Design review of the part built by this model. Coordinates are the model's own, in mm. Face numbers are marked on the shaded views. A direction names the side the tool comes from. Coordinates: 2 decimals unless noted, no trailing zeros. Write each loop counter-clockwise with the first axis right and the second up, starting at its lowest first coordinate (ties: lowest second). Pieces come first, ordered by that corner, then holes.
Q1. Take a section at D-D, the plane x = 7. Write out the cut boundary in (y, z), plus the area to 3 significant figures.
Q2. Take a section at C-C, the plane y = 207. Write out the cut boundary in (x, z), plus the area to 3 significant figures.
Q3. Take a section at B-B, the plane x = 63. Write out the cut boundary in (y, z), plus the area to 3 significant figures.
Q4. For the marked faces 1 and 2, list the 3-axis set-ups (+Z, -Z, +X, -X, +Y, -Y) from which the entire face can be reached by the end or side of a thin tool; tool diameter is ignored.
Q5. For L1, parallel to Y at x = 87, z = -179.5; L2, parallel to Y at x = 46, z = -109; L3, parallel to X at y = 98, z = -88, list the stretches that pass through material, from the lowest coordinate up.
Q6. The part is to be moulded in two halves that separate along Y. For the marked faces 3, 4 and 5, say which applies: released by +Y, released by -Y, zero draft, split by the parting line, or undercut.
Q7. Take a section at A-A, the plane y = 36. Write out the cut boundary in (x, z).
Q8. For pin 1 Ø2 at (x, y) = (40, 225) entering from -Z; pin 2 Ø4 at (x, y) = (127.5, 58.5) entering from -Z; pin 3 Ø8 at (x, y) = (155, 320.5) entering from +Z, all flat-tipped, find the tip position at first contact; note any pin that passes through.
from build123d import *

# Parameters (mm, degrees)
BOSS_EXTRUDE1_DEPTH      = 254
BOSS_EXTRUDE2_DEPTH      = 165.1
BOSS_EXTRUDE2_DEPTH_BACK = 50.8
SKETCH16_R               = 20.3962
SKETCH17_R               = 25.4762
BOSS_EXTRUDE3_DEPTH      = 10.16
FILLET1_R                = 2.54
CUT_EXTRUDE5_DEPTH       = 518.859576594
CUT_EXTRUDE14_DEPTH      = 516.224718622
CUT_EXTRUDE16_DEPTH      = 488.341428789


with BuildPart() as part:
    # Sketch2 → Boss-Extrude1 (new body)
    with BuildSketch(Plane(origin=(0, 0, 0), x_dir=(1, 0, 0), z_dir=(0, 1, 0))):
        Polygon((0, 0), (130.302, 0), (154.729351402, 205.052140948), (-52.123869843, 143.209155408), align=None)
    extrude(amount=BOSS_EXTRUDE1_DEPTH)

    # Sketch16 → Boss-Extrude2 (add, two sides: drawn at the far end of the back side and taken through both)
    with BuildSketch(Plane(origin=(141.332693429, 246.526276938, 16.836612147), x_dir=(0.11829111292954252, 0, -0.9929789587911166), z_dir=(0.4964894793955593, 0.8660254037844382, 0.059145556464771376)).offset(-BOSS_EXTRUDE2_DEPTH_BACK)):
        with Locations(Location((59.539258978, 48.389402794, 0), (0, 0, 95.890220986))):
            Circle(SKETCH16_R)
    extrude(amount=BOSS_EXTRUDE2_DEPTH + BOSS_EXTRUDE2_DEPTH_BACK)

    # Sketch17 → Boss-Extrude3 (add)
    with BuildSketch(Plane(origin=(223.303106477, 389.507071103, 26.601543519), x_dir=(0.8680427390684899, -0.49533563558134813, -0.0338291482851031), z_dir=(0.49648947939555943, 0.866025403784438, 0.0591455564647714))):
        with Locations(Location((-39.824375463, 65.578020566, 0), (0, 0, 178.057961601))):
            Circle(SKETCH17_R)
    extrude(amount=-BOSS_EXTRUDE3_DEPTH)

    # Fillet1
    fillet1_edges = [part.edges().sort_by_distance(p)[0] for p in [
        (201.384117467, 394.758696828, -38.077767579),
        (210.835574876, 401.03092525, -37.476848726),
    ]]
    fillet(fillet1_edges, radius=FILLET1_R)

    # Sketch37 → Cut-Extrude5 (cut, through all)
    with BuildSketch(Plane(origin=(-74.235573647, 46.74358774, 4.634969946), x_dir=(0.044647299319108304, -0.028112868945999136, 0.9986071726475507), z_dir=(-0.8450404746161061, 0.5320929256471292, 0.052760920546034554))):
        Polygon((-177.193506747, 239.03382897), (-117.503506747, 239.03382897), (-4.641434663, 139.710775348), (-148.050333908, 53.903642677), align=None)
    extrude(amount=CUT_EXTRUDE5_DEPTH, mode=Mode.SUBTRACT)

    # Sketch44 → Cut-Extrude14 (cut, through all)
    with BuildSketch(Plane(origin=(-77.674407605, 59.476403537, 15.773333495), x_dir=(-0.1263811849383747, 0.0967718787528128, -0.9872502213604327), z_dir=(0.7838483769002791, -0.6002039000265006, -0.1591760045477231))):
        Polygon((129.968891102, 229.15973728), (15.977037182, 243.05344524), (15.977037182, 131.08466752), align=None)
    extrude(amount=-CUT_EXTRUDE14_DEPTH, mode=Mode.SUBTRACT)


with BuildPart() as cut_extrude14_piece_1:
    # of the separate pieces the step leaves, piece 1, a body of its own (cut_extrude14_pieces)
    add(part.part.solids().sort_by_distance((164.733826071, 412.847507441, -38.227997293))[0])


with BuildPart() as cut_extrude14_piece_2:
    # of the separate pieces the step leaves, piece 2, a body of its own (cut_extrude14_pieces)
    add(part.part.solids().sort_by_distance((-24.451989708, 254, -67.181289582))[0])

    # Sketch54 → Cut-Extrude16 (cut, through all)
    with BuildSketch(Plane(origin=(48.324107263, 47.921039084, 57.272316376), x_dir=(0.8395487608428681, -0.34863488518909047, -0.4166672473286021), z_dir=(0.5432843437530708, 0.5387528450113599, 0.6438846898513436))):
        Polygon((-57.559619545, 126.622022749), (-3.698754498, 267.020987435), (-89.385563224, 299.892779983), (-143.246428271, 159.493815297), align=None)
    extrude(amount=-CUT_EXTRUDE16_DEPTH, mode=Mode.SUBTRACT)


solid = cut_extrude14_piece_1.part
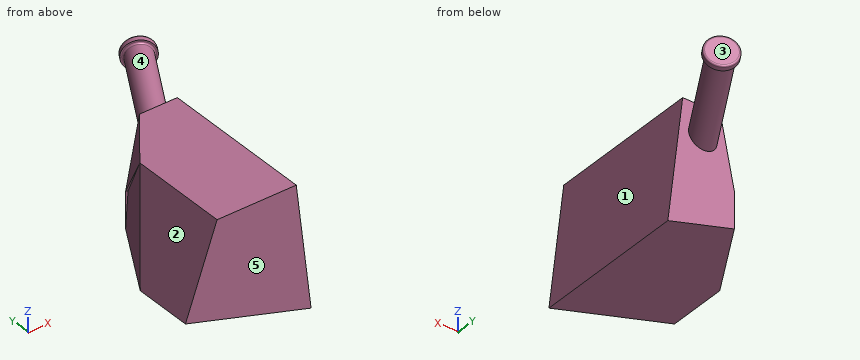
Responses:
1. outline: (0, -160.89) - (192.17, -160.89) - (177.85, -16.48) - (178.86, -17.42) - (174.24, 0) - (0, 0) - close
1. area: 29,600 mm2
2. outline: (16.17, -163.63) - (154.73, -205.05) - (130.3, 0) - (32.08, 0) - (21.31, -53.04) - (23, -54.14) - close
2. area: 22,100 mm2
3. outline: (0, -177.63) - (254, -177.63) - (254, -24.98) - (247.38, 0) - (0, 0) - close
3. area: 45,000 mm2
4. face 1: +Z, +X, -Y
4. face 2: +Z, -X, +Y, -Y
5. L1: y = 0 to 254
5. L2: y = 0 to 248.96, 249.67 to 254
5. L3: x = -32.03 to 140.79
6. face 3: released by +Y
6. face 4: undercut
6. face 5: released by -Y
7. outline: (-52.12, -143.21) - (154.73, -205.05) - (130.3, 0) - (0, 0) - close
8. pin 1: stops at z = -171.05
8. pin 2: stops at z = -197.51
8. pin 3: stops at z = -27.58
